Input: part model. Units: mm. Frame: model coordinates. Face numbers are marked on the shaded views. A direction names the side the tool comes from. Round coordinates to 2 decimals unless told otherwise and drop trailing zeros. Loops run counter-clockwise (first coordinate to the right, second up) from the corner with the lowest first, then second, coordinate; pieces in that order, holes last. Notation, with made-up numbers: (13, 50.5) -> (39, 50.5) arc R23 ccw to (39, 63.5) -> close; hole circle Ø5 at (80.25, 53.5). An arc over 180 degrees is marked (long way). Answer as a JSON object with one key per item and string values. Group by question number.
Item 1: Section query C-C on x = 0.6. Return loops of the section in (y, z), and give its area (3 significant figures).
Item 2: Material intervals for line 1 (Y direction, x = 0.6, z = 2.75); line 2 (Z direction, x = -3.25, y = -2.75); line 3 (Y direction, x = 1, z = 7.75), sorted ascending. Write a range as [from, to].
Item 3: Section query D-D on y = 4.25. Return loops of the section in (x, z), and give its area (3 significant figures).
Item 4: Set-up query: the marked faces 4, 5 and 6. Return all of +Z, -Z, +X, -X, +Y, -Y with unobstructed straight access to the full face (end or side cutting, diameter ignored); none if empty.
Item 5: Pin query (flat end, axial travel): pin 1 (1.4 mm diameter, centred on y = -0.5, z = 3, fed in from -X) (3 decimals); pin 2 (1.5 mm diameter, centred on y = -1, z = 7, fed in from -X); pin 3 (1 mm diameter, centred on y = -3.5, z = 1.5, fed in from +X). Return the tip coordinate at first contact, or that it passes through.
Item 6: Section query A-A on y = 0. Return loops of the section in (x, z) (3 decimals), and give its area (3 significant figures).
Item 7: Draft query along X for the marked faces 1, 2 and 3. Return one class per face: released by +X, released by -X, zero draft, split by the parting line, or undercut.
Item 8: Section query B-B on z = 2.25. Return loops of the section in (x, y) (3 decimals), and give its area (3 significant figures).
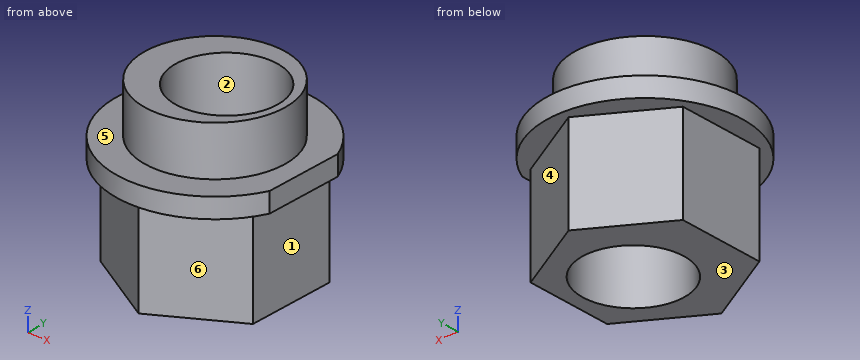
from build123d import *

# Parameters (mm, degrees)
F1_DEPTH  = 5
F2_R      = 3.575
F3_DEPTH  = 3.5
F4_R      = 2.6
F5_DEPTH  = 25
F6_R      = 5
F7_DEPTH  = 1
F8_R      = 2.6
F9_DEPTH  = 25
F10_W     = 1.5
F10_H     = 5
F11_DEPTH = 2


with BuildPart() as f1:
    # F0 (on Top) → F1 (new body)
    with BuildSketch(Plane.XY):
        Polygon((3.925, -2.2661), (3.925, 2.2661), (0, 4.5322), (-3.925, 2.2661), (-3.925, -2.2661), (0, -4.5322), align=None)
    extrude(amount=F1_DEPTH)

    # F2 (on face) → F3 (join)
    with BuildSketch(Plane.XY.offset(5)):
        Circle(F2_R)
    extrude(amount=F3_DEPTH)

    # F4 (on face) → F5 (cut)
    with BuildSketch(Plane.XY.offset(8.5)):
        with Locations((0.6, 0)):
            Circle(F4_R)
    extrude(amount=-F5_DEPTH, mode=Mode.SUBTRACT)

    # F6 (on face) → F7 (join)
    with BuildSketch(Plane.XY.offset(5)):
        Circle(F6_R)
    extrude(amount=F7_DEPTH)

    # F8 (on face) → F9 (cut)
    with BuildSketch(Plane.XY.offset(8.5)):
        with Locations((0.6, 0)):
            Circle(F8_R)
    extrude(amount=-F9_DEPTH, mode=Mode.SUBTRACT)

    # F10 (on face) → F11 (cut)
    with BuildSketch(Plane.XY.offset(6)):
        with Locations((5.325, 0)):
            Rectangle(F10_W, F10_H)
    extrude(amount=-F11_DEPTH, mode=Mode.SUBTRACT)


solid = f1.part
Solved:
{
 "1": {"outline": "(-4.96, 5) -> (-4.19, 5) -> (-4.19, 0) -> (-2.6, 0) -> (-2.6, 8.5) -> (-3.52, 8.5) -> (-3.52, 6) -> (-4.96, 6) -> close; (2.6, 0) -> (4.19, 0) -> (4.19, 5) -> (4.96, 5) -> (4.96, 6) -> (3.52, 6) -> (3.52, 8.5) -> (2.6, 8.5) -> close", "area": "25.2 mm²"},
 "2": {"line 1": "[-4.19, -2.6], [2.6, 4.19]", "line 2": "[5, 6]", "line 3": "[-3.43, -2.57], [2.57, 3.43]"},
 "3": {"outline": "(-2.63, 5) -> (-0.49, 5) -> (-0.49, 0) -> (0.49, 0) -> (0.49, 5) -> (2.63, 5) -> (2.63, 6) -> (-2.63, 6) -> close", "area": "10.2 mm²"},
 "4": {"face 4": "-Z, +X, +Y", "face 5": "+Z", "face 6": "-Z, +X, -Y"},
 "5": {"pin 1": "x = -3.925", "pin 2": "x = -3.57", "pin 3": "x = 2.65"},
 "6": {"outline": "(-5, 5) -> (-3.925, 5) -> (-3.925, 0) -> (-2, 0) -> (-2, 8.5) -> (-3.575, 8.5) -> (-3.575, 6) -> (-5, 6) -> close; (3.2, 0) -> (3.925, 0) -> (3.925, 5) -> (4.575, 5) -> (4.575, 6) -> (3.575, 6) -> (3.575, 8.5) -> (3.2, 8.5) -> close", "area": "22.5 mm²"},
 "7": {"face 1": "released by +X", "face 2": "undercut", "face 3": "zero draft"},
 "8": {"outline": "(-3.925, -2.266) -> (0, -4.532) -> (3.925, -2.266) -> (3.925, 2.266) -> (0, 4.532) -> (-3.925, 2.266) -> close; hole circle Ø5.2 at (0.6, 0)", "area": "32.1 mm²"}
}
